```python
from build123d import *

# Parameters (mm, degrees)
SKETCH1_W           = 25
SKETCH1_H           = 25
BOSS_EXTRUDE1_DEPTH = 33.74
SKETCH2_R           = 9.525
CUT_EXTRUDE1_DEPTH  = 30
SKETCH3_W           = 12.5
SKETCH3_H           = 25
CUT_EXTRUDE2_DEPTH  = 39.090518505
SKETCH4_R           = 2.5
CUT_EXTRUDE3_DEPTH  = 39.090518505
CHAMFER2_SIZE       = 0.5
FILLET1_R           = 1


with BuildPart() as part:
    # Sketch1 → Boss-Extrude1 (new body)
    with BuildSketch(Plane(origin=(0, 0, 0), x_dir=(1, 0, 0), z_dir=(0, 1, 0))):
        Rectangle(SKETCH1_W, SKETCH1_H)
    extrude(amount=BOSS_EXTRUDE1_DEPTH)

    # Sketch2 → Cut-Extrude1 (cut)
    with BuildSketch(Plane(origin=(0, 33.74, 0), x_dir=(1, 0, 0), z_dir=(0, 1, 0))):
        with Locations(Location((0, 0, 0), (0, 0, 270))):
            Circle(SKETCH2_R)
    extrude(amount=-CUT_EXTRUDE1_DEPTH, mode=Mode.SUBTRACT)

    # Sketch3 → Cut-Extrude2 (cut, through all)
    with BuildSketch(Plane(origin=(0, 33.74, 0), x_dir=(1, 0, 0), z_dir=(0, 1, 0))):
        with Locations((6.25, 0)):
            Rectangle(SKETCH3_W, SKETCH3_H)
    extrude(amount=-CUT_EXTRUDE2_DEPTH, mode=Mode.SUBTRACT)

    # Sketch4 → Cut-Extrude3 (cut, through all)
    with BuildSketch(Plane.ZY.offset(12.5)):
        with Locations((0, 27.74)):
            Circle(SKETCH4_R)
        with Locations((0, 9.74)):
            Circle(SKETCH4_R)
    extrude(amount=-CUT_EXTRUDE3_DEPTH, mode=Mode.SUBTRACT)

    # Chamfer2
    chamfer2_edges = [part.edges().sort_by_distance(p)[0] for p in [
        (-12.5, 33.74, 0),
        (-6.25, 33.74, 12.5),
        (-6.25, 0, -12.5),
        (-6.25, 33.74, -12.5),
        (-6.25, 0, 12.5),
        (-12.5, 0, 0),
        (-12.5, 16.87, 12.5),
        (-12.5, 16.87, -12.5),
    ]]
    chamfer(chamfer2_edges, length=CHAMFER2_SIZE)

    # Fillet1
    fillet1_edges = [part.edges().sort_by_distance(p)[0] for p in [
        (-9.525, 33.74, 0),
        (0, 18.74, 9.525),
        (0, 18.74, -9.525),
    ]]
    fillet(fillet1_edges, radius=FILLET1_R)


solid = part.part
```
The listing builds one solid part. Answer for the finished solid, in the listing's coordinates (mm). A direction names the side the tool comes from. Coordinates: 2 decimals unless noted, no trailing zeros. Write each loop counter-clockwise with the first axis right and the second up, starting at its lowest first coordinate (ties: lowest second). Pieces come first, ordered by that corner, then holes. Notation, with made-up numbers: M 86.5,41.25 L 126.5,41.25 A34 cw 126.5,79.25 Z; hole C 84.5,74.5 d10. An arc over 180 degrees is marked long. Use a Markdown table: item, result. Add a question column.
1. Section A-A (y = 27.74) is taken. Give the vertices of the cut face in (x, z) (3 decimals), plus the area to 3 significant figures.
2. Section B-B (z = 0) is taken. Give the vertices of the cut face in (x, y) (3 decimals), plus the area to 3 significant figures.
3. Which of the six approach directions +Z, -Z, +X, -X, +Y, -Y give full straight-line access (tool end or side, diameter ignored) to faces 5 (the flat face through (-6, 17, -12.5)), 6 (the cylindrical face through (-9.523, 18.443, -0.197))?
4. For a pull along Z with two mould halves and no side action, classify faces 1 (the flat face through (-4, 3.74, 0)), 2 (the cylindrical face through (-10.9, 9.8, -2.5)), 3 (the flat face through (-11, 33.74, 0)), 4 (the flat face through (-6, 17, 12.5)) as +Z half, -Z half, draft (parallel to the pull), parting line (faces both ways), or undercut.
5. Given P1, Ø2, axis at y = 29.5, z = 3.5, coming from the +X side (3 decimals); P2, Ø4, axis at y = 9.74, z = 0, coming from the +X side; P3, Ø6, axis at y = 23, z = -5.5, coming from the +X side; P4, Ø3, axis at x = -4, z = -1.5, coming from the +Y side, each flat-ended and moving along its own axis, determine where each tip first touches the part or whether it passes through.
6. Section C-C (y = 10.5) is taken. Give the vertices of the cut face in (x, z) (3 decimals).
7. Straight lines are drawn through the part: line 1 along Y through (x, z) = (-11.1, 0); line 2 along Z through (x, y) = (-10.2, 9.74); line 3 along Y through (x, z) = (-8, -5). For each, find the intervals that lie inside material, in ascending order. Write a range as [from, to].
Data:
| question | item | result |
|---|---|---|
| 1 | outline | M -12.5,-12 L -12,-12.5 L 0,-12.5 L 0,-10.477 A1 ccw -0.905,-9.482 A9.525 cw -9.191,-2.5 L -12.5,-2.5 Z; M -12.5,2.5 L -9.191,2.5 A9.525 cw -0.905,9.482 A1 ccw 0,10.477 L 0,12.5 L -12,12.5 L -12.5,12 Z |
| 1 | area | 154 mm2 |
| 2 | outline | M -12.5,0.5 L -12,0 L 0,0 L 0,3.74 L -9.525,3.74 L -9.525,7.24 L -12.5,7.24 Z; M -12.5,12.24 L -9.525,12.24 L -9.525,25.24 L -12.5,25.24 Z; M -12.5,30.24 L -9.525,30.24 L -9.525,32.74 A1 ccw -10.525,33.74 L -12,33.74 L -12.5,33.24 Z |
| 2 | area | 106 mm2 |
| 3 | face 5 | -Z, +X, -X, +Y, -Y |
| 3 | face 6 | +X, +Y |
| 4 | face 1 | undercut |
| 4 | face 2 | undercut |
| 4 | face 3 | draft |
| 4 | face 4 | +Z half |
| 5 | P1 | stops at x = -8.395 |
| 5 | P2 | passes through |
| 5 | P3 | stops at x = -4.3 |
| 5 | P4 | stops at y = 3.74 |
| 6 | outline | M -12.5,-12 L -12,-12.5 L 0,-12.5 L 0,-10.477 A1 ccw -0.905,-9.482 A9.525 cw -9.222,-2.382 L -12.5,-2.382 Z; M -12.5,2.382 L -9.222,2.382 A9.525 cw -0.905,9.482 A1 ccw 0,10.477 L 0,12.5 L -12,12.5 L -12.5,12 Z |
| 7 | line 1 | y = [0, 7.24], [12.24, 25.24], [30.24, 33.74] |
| 7 | line 2 | z = [-12.5, -2.5], [2.5, 12.5] |
| 7 | line 3 | y = [0, 3.74] |
